```python
from build123d import *

# Parameters (mm, degrees)
F1_DEPTH = 24
F2_W     = 99.111150098
F2_H     = 9
F2_W_2   = 5.3233464885


with BuildPart() as f1:
    # F0 (on Front) → F1 (new body, symmetric)
    with BuildSketch(Plane.XZ):
        Polygon((-28.5438378341, 48), (-28.5438378341, 0), (67.4561621659, 0), (67.6174540565, 23.9994580132), align=None)
    extrude(amount=F1_DEPTH, both=True)

    # F2 (on face) → F3 (revolve, cut)
    with BuildSketch(Plane(origin=(9.6037996504, 0, 38.4788719333), x_dir=(0.9702368684, 0, -0.2421578396), z_dir=(0.2421578396, 0, 0.9702368684))):
        with Locations((10.2377149176, 4.5)):
            Rectangle(F2_W, F2_H)
        with Locations((62.4549632108, 4.5)):
            Rectangle(F2_W_2, F2_H)
    revolve(axis=Axis((22.1192616243, 0, 35.3551839641), (0.9702368684, 0, -0.2421578396)), mode=Mode.SUBTRACT)


solid = f1.part
```
Source: CAD feature listing. Evaluate the final solid. Frame: model axes, mm. Give positions to 0.01 mm unless a question says otherwise; leave off trailing zeros. Loops run counter-clockwise (first coordinate to the right, second up) from the corner with the lowest first, then second, coordinate; pieces in that order, holes last. Notation, with made-up numbers: (17.25, 29) -> (31.25, 29) arc R22 ccw to (31.25, 44) -> close; hole circle Ø6 at (-20, -29). An arc over 180 degrees is marked (long way). Use a Markdown table: item, result. Add a question column.
(1) Pull-direction query (Y, two-part tool) for faces 1 (the face through (17.75, -0.2, 27.17)), 2 (the face through (-28.544, 0, 24)), 3 (the face through (19, -24, 19)); classes: +Y half, -Y half, draft (parallel to the pull), parting line (faces both ways), or undercut.
(2) Section query A-A (y = -21). Output: boundary loops of the cut face in (x, z).
(3) First-contact query: pin 1 Ø6 at (x, y) = (10, -8) entering from +Z; pin 2 Ø12 at (y, z) = (-8.5, 8) entering from +X; pin 3 Ø3 at (y, z) = (16.5, 10) entering from +X. Flat tips, straight axial feed; report the tip coordinate or a pass-through.
(4) Section query B-B (y = 2). Output: boundary loops of the cut face in (x, z).
(5) Ray query, line 1 (X direction, y = 9, z = 12); line 2 (Z direction, x = -4.5, y = 5); line 3 (Z direction, x = 62, y = -13). Return the intervals inside material, ascending.
Checked values:
| question | item | result |
|---|---|---|
| 1 | face 1 | undercut |
| 1 | face 2 | draft |
| 1 | face 3 | -Y half |
| 2 | outline | (-28.54, 0) -> (67.46, 0) -> (67.62, 24) -> (-28.54, 48) -> close |
| 3 | pin 1 | z = 39.09 |
| 3 | pin 2 | x = 67.55 |
| 3 | pin 3 | x = 67.53 |
| 4 | outline | (-28.54, 0) -> (67.46, 0) -> (67.56, 14.97) -> (-28.54, 38.96) -> close |
| 5 | line 1 | -28.54 to 67.54 |
| 5 | line 2 | 0 to 34.29 |
| 5 | line 3 | 0 to 25.4 |
